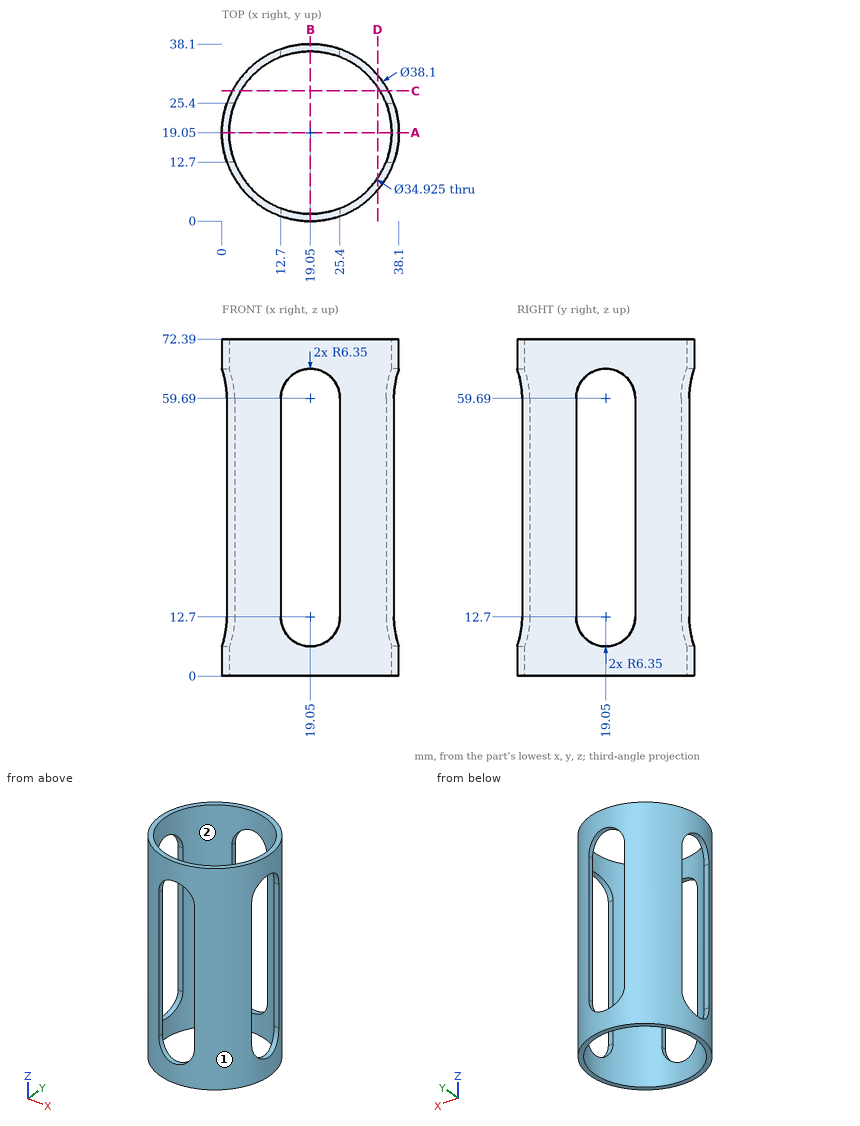
The figure shows three views and two pictorial views of one solid part (mm, origin at its lowest corner). Answer the questions. Coordinates: 2 decimals unless noted, no trailing zeros. Loops run counter-clockwise (first coordinate to the right, second up) from the corner with the lowest first, then second, coordinate; pieces in that order, holes last. Notation, with made-up numbers: (78.5, 8) -> (125.5, 8) arc R34 ccw to (125.5, 44) -> close; hole circle Ø8 at (85.25, -39). An arc over 180 degrees is marked (long way). Return JSON: item names as keys, results as strings. Group by question number.
(1) A cutting plane is placed at D-D on x = 33.5. Write down the section's boundary in (y, z), and give its area (3 significant figures).
(2) A cutting plane is placed at C-C on y = 28. Write down the section's boundary in (x, z), and give its area (3 significant figures).
(3) A cutting plane is placed at A-A on y = 19.05. Write down the section's boundary in (x, z).
(4) Find the intervals of material crossed by probe 1 along X at (y, z) = (5, 43); probe 2 along Y at (x, z) = (5.5, 12.5); probe 3 along X at (y, z) = (26.5, 35), in increasing order. Write a range as from..to.
(5) Determine the mould class of the marked faces 1 and 2 for opening direction X: released by +X, released by -X, zero draft, split by the parting line, or undercut.
(6) Given pin 1 Ø2 at (x, z) = (28, 24.5) entering from -Y; pin 2 Ø0.8 at (y, z) = (36.5, 39.5) entering from +X; pin 3 Ø1.4 at (x, z) = (36, 27) entering from -Y, each flat-ended and moving along its own axis, determine where each tip first touches the part or whether it passes through.
The answers:
{
 "1": {"outline": "(6.64, 0) -> (9.25, 0) -> (9.25, 72.39) -> (6.64, 72.39) -> close; (28.85, 0) -> (31.46, 0) -> (31.46, 72.39) -> (28.85, 72.39) -> close", "area": "378 mm^2"},
 "2": {"outline": "(2.23, 0) -> (4.06, 0) -> (4.06, 72.39) -> (2.23, 72.39) -> close; (34.04, 0) -> (35.87, 0) -> (35.87, 72.39) -> (34.04, 72.39) -> close", "area": "264 mm^2"},
 "3": {"outline": "(0, 0) -> (1.59, 0) -> (1.59, 6.35) -> (0, 6.35) -> close; (0, 66.04) -> (1.59, 66.04) -> (1.59, 72.39) -> (0, 72.39) -> close; (36.51, 0) -> (38.1, 0) -> (38.1, 6.35) -> (36.51, 6.35) -> close; (36.51, 66.04) -> (38.1, 66.04) -> (38.1, 72.39) -> (36.51, 72.39) -> close"},
 "4": {"probe 1": "x = 6.19..8.68, 29.42..31.91", "probe 2": "y = 5.66..8.03, 30.07..32.44", "probe 3": "x = 1.52..3.26, 34.84..36.58"},
 "5": {"face 1": "split by the parting line", "face 2": "undercut"},
 "6": {"pin 1": "stops at y = 1.74", "pin 2": "stops at x = 27.55", "pin 3": "stops at y = 9.11"}
}
